Answer from the drawing. Dimensions are ordinates in mm from the lowest x, y and z of the part. A direction names the side the tool comes from. Coordinates: 2 decimals unless noted, no trailing zeros. Loops run counter-clockwise (first coordinate to the right, second up) from the corner with the lowest first, then second, coordinate; pieces in that order, holes last.
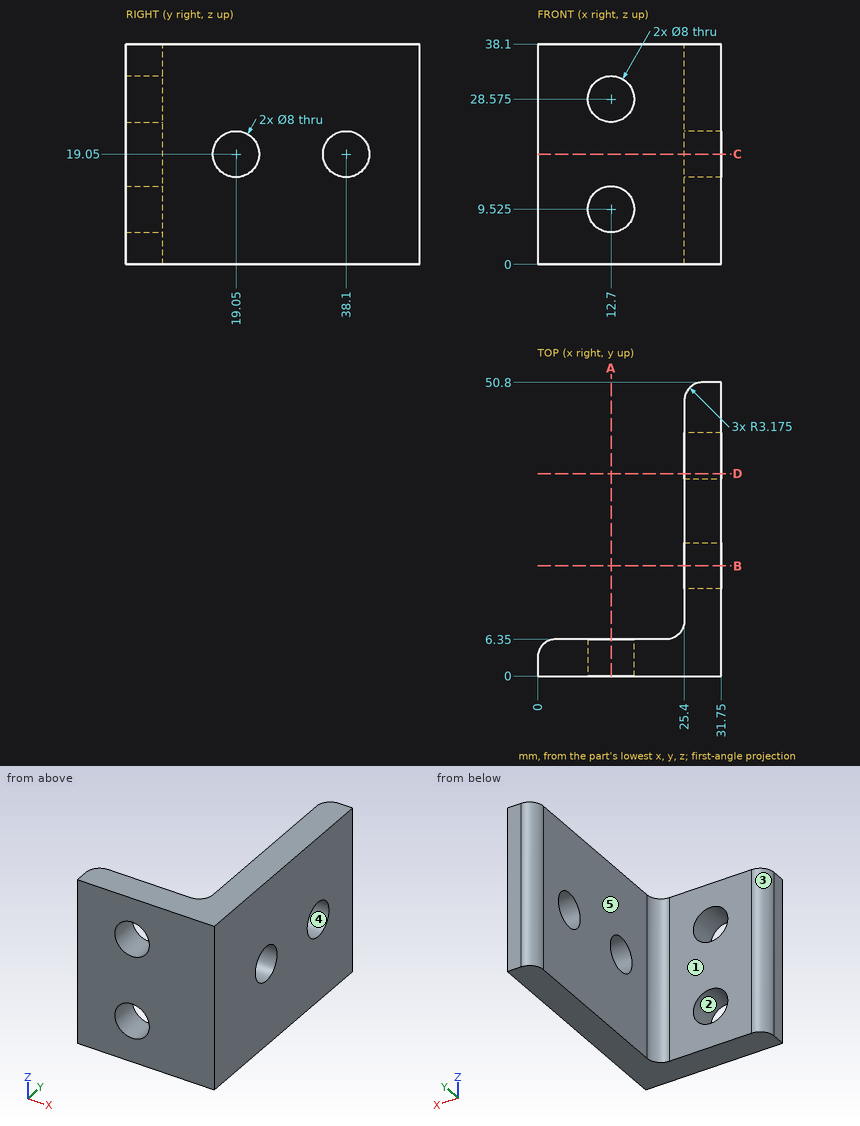
Item 1: A cutting plane is placed at B-B on y = 19.05. Determine the outline of the cut face in (x, z).
Numbers:
outline: (25.4, 0) - (31.75, 0) - (31.75, 15.05) - (25.4, 15.05) - close; (25.4, 23.05) - (31.75, 23.05) - (31.75, 38.1) - (25.4, 38.1) - close
Item 2: A cutting plane is placed at C-C on z = 19.05. Determine the outline of the cut face in (x, y) (3 decimals), then the cut area to 3 significant figures.
Numbers:
outline: (0, 0) - (31.75, 0) - (31.75, 15.05) - (25.4, 15.05) - (25.4, 9.525) arc R3.175 cw to (22.225, 6.35) - (3.175, 6.35) arc R3.175 ccw to (0, 3.175) - close; (25.4, 23.05) - (31.75, 23.05) - (31.75, 34.1) - (25.4, 34.1) - close; (25.4, 42.1) - (31.75, 42.1) - (31.75, 50.8) - (28.575, 50.8) arc R3.175 ccw to (25.4, 47.625) - close
area: 380 mm2
Item 3: Determine the mould class of the marked faces 1, 2 and 3 for opening direction X: released by +X, released by -X, zero draft, split by the parting line, or undercut.
Numbers:
face 1: zero draft
face 2: undercut
face 3: released by -X
Item 4: A cutting plane is placed at A-A on x = 12.7. Determine the outline of the cut face in (y, z) (3 decimals).
Numbers:
outline: (0, 0) - (6.35, 0) - (6.35, 5.525) - (0, 5.525) - close; (0, 13.525) - (6.35, 13.525) - (6.35, 24.575) - (0, 24.575) - close; (0, 32.575) - (6.35, 32.575) - (6.35, 38.1) - (0, 38.1) - close
Item 5: Given pin 1 (1 mm diameter, centred on y = 20.5, z = 14.5, fed in from -X); pin 2 (8 mm diameter, centred on x = 25, y = 28.5, fed in from +Z); pin 3 (2 mm diameter, centred on x = 25.5, z = 33, fed in from +Y), each flat-ended and moving along its own axis, determine where each tip first touches the part or whether it passes through.
Numbers:
pin 1: stops at x = 25.4
pin 2: stops at z = 38.1
pin 3: stops at y = 50.03
Item 6: A cutting plane is placed at D-D on y = 35. Determine the outline of the cut face in (x, z).
Numbers:
outline: (25.4, 0) - (31.75, 0) - (31.75, 16.52) - (25.4, 16.52) - close; (25.4, 21.58) - (31.75, 21.58) - (31.75, 38.1) - (25.4, 38.1) - close
Item 7: Find the intervals of material crossed by line 1 along Z through (x, y) = (12.7, 4.75) (3 decimals); line 2 along Y through (x, z) = (27, 19); line 3 along Z through (x, y) = (28.5, 38.1), in increasing order.
Numbers:
line 1: z = 0 to 5.525, 13.525 to 24.575, 32.575 to 38.1
line 2: y = 0 to 15.05, 23.05 to 34.1, 42.1 to 50.38
line 3: z = 0 to 15.05, 23.05 to 38.1
Item 8: Which of the six approach directions +Z, -Z, +X, -X, +Y, -Y give full straight-line access (tool end or side, diameter ignored) to the marked faces 4 and 5?
Numbers:
face 4: +X, -X
face 5: +Z, -Z, -X, +Y
